The listing builds one solid part. Answer for the finished solid, in the listing's coordinates (mm). A direction names the side the tool comes from. Coordinates: 2 decimals unless noted, no trailing zeros. Write each loop counter-clockwise with the first axis right and the second up, starting at its lowest first coordinate (ties: lowest second). Pieces come first, ordered by that corner, then holes.
(1) For a pull along X with two mould halves and no side action, classify faces 1 (the flat face through (-2.174, -4, 11)), 2 (the flat face through (-2.174, -4, -11)), 3 (the flat face through (-2.33, -5.83, -8)), 4 (the flat face through (2, 0, 0)) as +X half, -X half, draft (parallel to the pull), parting line (faces both ways), or undercut.
(2) The part is cut by section B-B on x = -2.75. Determine the outline of the cut face in (y, z), plus the area to 3 significant figures.
(3) Given P1, Ø0.8, axis at x = -3, z = -11, coming from the +Y side; P2, Ø2, axis at x = 0, z = 5.5, coming from the -Y side; P3, Ø6, axis at y = -5, z = 2.5, coming from the -X side, each flat-ended and moving along its own axis, determine where each tip first touches the part or whether it passes through.
(4) Which of the six approach directions +Z, -Z, +X, -X, +Y, -Y give full straight-line access (tool end or side, diameter ignored) to faces 5 (the flat face through (1, -6.5, 0)), 6 (the flat face through (-4, -1.5, 12)), 7 (the cylindrical face through (2.03, 0.9, -12.45))?
(5) The part is cut by section D-D on x = 3. Determine the outline of the cut face in (y, z).
(6) Straight lines are drawn through the part: line 1 (Z direction, x = -3.5, y = -7); line 2 (Z direction, x = 1.5, y = -1.25); line 3 (X direction, y = -2.5, z = 10). For each, find the intervals that lie inside material, in ascending order.
(7) The part is cut by section A-A on y = 0. Determine the outline of the cut face in (x, z).
(8) The part is cut by section C-C on x = 1.5. Determine the outline of the cut face in (y, z).
from build123d import *

# Parameters (mm, degrees)
ESQUISSE1_W             = 30
ESQUISSE1_H             = 17
BOSS_EXTRU_1_DEPTH      = 2
ESQUISSE2_R             = 5
BOSS_EXTRU_2_DEPTH      = 2
ESQUISSE3_R             = 3
ENL_V_MAT_EXTRU_1_DEPTH = 18.69887002
ESQUISSE4_R             = 3
ENL_V_MAT_EXTRU_2_DEPTH = 18.69887002
ESQUISSE7_W             = 2
ESQUISSE7_H             = 8
ENL_V_MAT_EXTRU_3_DEPTH = 2
ESQUISSE8_W             = 7
ESQUISSE8_H             = 2
BOSS_EXTRU_3_DEPTH      = 5
ESQUISSE12_W            = 2.825864409
ESQUISSE12_H            = 7
BOSS_EXTRU_4_DEPTH      = 5


with BuildPart() as part:
    # Esquisse1 → Boss.-Extru.1 (new body)
    with BuildSketch(Plane(origin=(0, 0, 0), x_dir=(0, 0, -1), z_dir=(1, 0, 0))):
        Rectangle(ESQUISSE1_W, ESQUISSE1_H)
    extrude(amount=BOSS_EXTRU_1_DEPTH)

    # Esquisse2 → Boss.-Extru.2 (add)
    with BuildSketch(Plane(origin=(2, 0, 0), x_dir=(0, 0, -1), z_dir=(1, 0, 0))):
        with Locations((-9.467846224, 0)):
            Circle(ESQUISSE2_R)
        with Locations((9.588622493, 0)):
            Circle(ESQUISSE2_R)
    extrude(amount=BOSS_EXTRU_2_DEPTH)

    # Esquisse3 → Enlèv. mat.-Extru.1 (cut, through all)
    with BuildSketch(Plane(origin=(4, 0, 0), x_dir=(0, 0, -1), z_dir=(1, 0, 0))):
        with Locations((-9.467846224, 0)):
            Circle(ESQUISSE3_R)
    extrude(amount=-ENL_V_MAT_EXTRU_1_DEPTH, mode=Mode.SUBTRACT)

    # Esquisse4 → Enlèv. mat.-Extru.2 (cut, through all)
    with BuildSketch(Plane(origin=(4, 0, 0), x_dir=(0, 0, -1), z_dir=(1, 0, 0))):
        with Locations((9.588622493, 0)):
            Circle(ESQUISSE4_R)
    extrude(amount=-ENL_V_MAT_EXTRU_2_DEPTH, mode=Mode.SUBTRACT)

    # Esquisse7 → Enlèv. mat.-Extru.3 (cut)
    with BuildSketch(Plane.XZ.offset(8.5)):
        with Locations((1, 4)):
            Rectangle(ESQUISSE7_W, ESQUISSE7_H)
    enl_v_mat_extru_3 = extrude(amount=-ENL_V_MAT_EXTRU_3_DEPTH, mode=Mode.SUBTRACT)

    # Symétrie1: Enlèv. mat.-Extru.3 across plane
    add(enl_v_mat_extru_3.mirror(Plane.XY), mode=Mode.SUBTRACT)

    # Esquisse8 → Boss.-Extru.3 (add)
    with BuildSketch(Plane.ZY):
        with Locations((-11.5, -7.5)):
            Rectangle(ESQUISSE8_W, ESQUISSE8_H)
    boss_extru_3 = extrude(amount=BOSS_EXTRU_3_DEPTH)

    # Esquisse12 → Boss.-Extru.4 (add)
    with BuildSketch(Plane(origin=(0, -6.5, 0), x_dir=(1, 0, 0), z_dir=(0, 1, 0))):
        with Locations((-3.587067796, 11.5)):
            Rectangle(ESQUISSE12_W, ESQUISSE12_H)
    boss_extru_4 = extrude(amount=BOSS_EXTRU_4_DEPTH)

    # Symétrie2: Boss.-Extru.3, Boss.-Extru.4 across plane
    add(boss_extru_3.mirror(Plane.XY))
    add(boss_extru_4.mirror(Plane.XY))


solid = part.part
Model answer:
1. face 1: undercut
1. face 2: undercut
1. face 3: draft
1. face 4: +X half
2. outline: (-8.5, -15) - (-1.5, -15) - (-1.5, -8) - (-8.5, -8) - close; (-8.5, 8) - (-1.5, 8) - (-1.5, 15) - (-8.5, 15) - close
2. area: 98.0 mm2
3. P1: stops at y = -1.5
3. P2: stops at y = -6.5
3. P3: stops at x = 0
4. face 5: +X, -X, -Y
4. face 6: +Z, -Z, -X, +Y
4. face 7: +X
5. outline: circle Ø10 at (0, -9.59); circle Ø10 at (0, 9.47); hole circle Ø6 at (0, -9.59); hole circle Ø6 at (0, 9.47)
6. line 1: z = -15 to -8, 8 to 15
6. line 2: z = -15 to -12.32, -6.86 to 6.74, 12.2 to 15
6. line 3: x = -5 to -2.17
7. outline: (0, -15) - (2, -15) - (2, -14.59) - (4, -14.59) - (4, -12.59) - (0, -12.59) - close; (0, -6.59) - (4, -6.59) - (4, -4.59) - (2, -4.59) - (2, 4.47) - (4, 4.47) - (4, 6.47) - (0, 6.47) - close; (0, 12.47) - (4, 12.47) - (4, 14.47) - (2, 14.47) - (2, 15) - (0, 15) - close
8. outline: (-8.5, -15) - (8.5, -15) - (8.5, 15) - (-8.5, 15) - (-8.5, 8) - (-6.5, 8) - (-6.5, -8) - (-8.5, -8) - close; hole circle Ø6 at (0, -9.59); hole circle Ø6 at (0, 9.47)
